from build123d import *

# Parameters (mm, degrees)
F0_R     = 1.925
F1_DEPTH = 1
F0_R_2   = 4.925
F2_DEPTH = 1.5
F3_SIZE  = 0.75
F4_T     = -0.7


with BuildPart() as f1:
    # F0 (on Top) → F1 (new body)
    with BuildSketch(Plane.XY):
        Circle(F0_R)
    extrude(amount=F1_DEPTH)

    # F0 (on Top) → F2 (join)
    with BuildSketch(Plane.XY):
        Circle(F0_R_2)
        Circle(F0_R, mode=Mode.SUBTRACT)
        Circle(F0_R)
    extrude(amount=-F2_DEPTH)

    # F3
    f3_edges = [f1.edges().sort_by_distance(p)[0] for p in [
        (-4.925, 0, 0),
    ]]
    chamfer(f3_edges, length=F3_SIZE)

    # F4
    f4_openings = [f1.faces().sort_by_distance(p)[0] for p in [
        (0, 0, 1),
    ]]
    offset(amount=F4_T, openings=f4_openings, kind=Kind.INTERSECTION)


solid = f1.part
Design review of the part built by this model. Coordinates are the model's own, in mm. A direction names the side the tool comes from. Round coordinates to 2 decimals unless told otherwise and drop trailing zeros. Write each loop counter-clockwise with the first axis right and the second up, starting at its lowest first coordinate (ties: lowest second). Pieces come first, ordered by that corner, then holes. Notation, with made-up numbers: M 46,62.5 L 102,62.5 A22 ccw 102,84.5 Z; hole C 12.25,-14.5 d10. An arc over 180 degrees is marked long. One line per item, written item: value. Start each with the question number.
1. Take a section at D-D on z = 0.4. State the section outline as (x, y) points (3 decimals).
2. To check wall thickness, follow probe 1 along Y at (x, z) = (0, 0.2) (3 decimals); probe 2 along Y at (x, z) = (-0.5, 0.75). State the ranges of each line that lie inside material, in increasing order. Write a range as from..to.
3. For faces 4 (the face through (2, -1, 0)), 5 (the face through (-3.908, -2.997, -1.12)), list the 3-axis set-ups (+Z, -Z, +X, -X, +Y, -Y) from which the entire face can be reached by the end or side of a thin tool; tool diameter is ignored.
4. Take a section at C-C on z = -1.25. State the section outline as (x, y) points (3 decimals), then the cut area to 3 significant figures.
5. Take a section at A-A on x = 0. State the section outline as (y, z) points (3 decimals).
6. Draft analysis for pull direction Y (two halves, no side actions). For faces 1 (the face through (0, 0, -0.8)), 2 (the face through (0, 0, -1.5)), 3 (the face through (-0.42, -1.88, 0.49)), state which applies: pulls with the +Y half, pulls with the -Y half, needs draft (parallel to the pull), parting line crosses it, or undercut.
Computed:
1. outline: C 0,0 d3.85; hole C 0,0 d2.45
2. probe 1: y = -1.925..-1.225, 1.225..1.925
2. probe 2: y = -1.86..-1.12, 1.12..1.86
3. face 4: +Z
3. face 5: +Z, -Z
4. outline: C 0,0 d9.85
4. area: 76.2 mm²
5. outline: M -4.925,-1.5 L 4.925,-1.5 L 4.925,-0.75 L 4.175,0 L 1.925,0 L 1.925,1 L 1.225,1 L 1.225,-0.7 L 3.885,-0.7 L 3.985,-0.8 L -3.985,-0.8 L -3.885,-0.7 L -1.225,-0.7 L -1.225,1 L -1.925,1 L -1.925,0 L -4.175,0 L -4.925,-0.75 Z
6. face 1: undercut
6. face 2: needs draft
6. face 3: parting line crosses it
